For this review, take the finished solid that the model builds, in its own axes (mm). Coordinates: 2 decimals unless noted, no trailing zeros. Write each loop counter-clockwise with the first axis right and the second up, starting at its lowest first coordinate (ties: lowest second). Pieces come first, ordered by that corner, then holes.
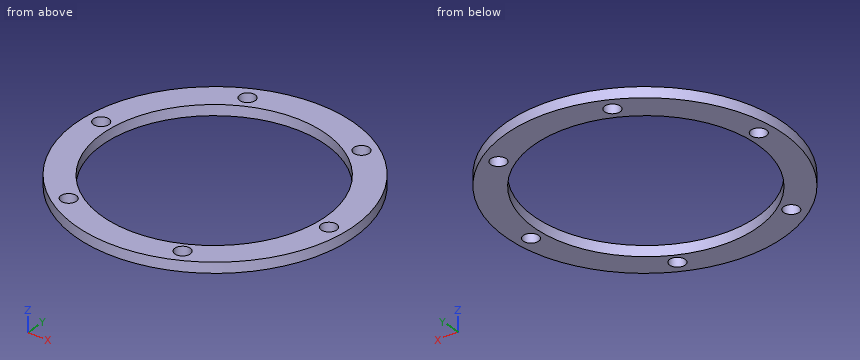
```python
from build123d import *

# Parameters (mm, degrees)
ESQUISSE1_R                  = 30.5
ESQUISSE1_R_2                = 24.5
BOSS_EXTRU_1_DEPTH           = 2.3
ENL_V_MAT_EXTRU_2_REACH      = 45.379
ESQUISSE1_3_R                = 1.7
R_P_TITION_CIRCULAIRE1_COUNT = 6


with BuildPart() as part:
    # Esquisse1 → Boss.-Extru.1 (new body)
    with BuildSketch(Plane.XY):
        with Locations((0, -0.260069897)):
            Circle(ESQUISSE1_R)
        with Locations((0, -0.525514899)):
            Circle(ESQUISSE1_R_2, mode=Mode.SUBTRACT)
    extrude(amount=BOSS_EXTRU_1_DEPTH)

    # Esquisse1_3 → Enl_v. mat.-Extru.2 (cut, up to next)
    with BuildSketch(Plane.XY, mode=Mode.PRIVATE) as enl_v_mat_extru_2_sk1:
        with Locations((15.543281325, 22.122264781)):
            Circle(ESQUISSE1_3_R)
    enl_v_mat_extru_2_tool1 = extrude(enl_v_mat_extru_2_sk1.sketch, amount=ENL_V_MAT_EXTRU_2_REACH, mode=Mode.PRIVATE) & part.part
    enl_v_mat_extru_2 = enl_v_mat_extru_2_tool1.solids().sort_by_distance((15.543281, 22.122265, 0))[0]
    add(enl_v_mat_extru_2, mode=Mode.SUBTRACT)

    # R_p_tition circulaire1: Enl_v. mat.-Extru.2 ×6 about axis
    r_p_tition_circulaire1_axis = Axis((0, -0.260069897, 0), (0, 0, 1))
    for i in range(1, R_P_TITION_CIRCULAIRE1_COUNT):
        add(enl_v_mat_extru_2.rotate(r_p_tition_circulaire1_axis, i * 360 / R_P_TITION_CIRCULAIRE1_COUNT), mode=Mode.SUBTRACT)


solid = part.part
```
Q1. For probe 1 along X at (y, z) = (2, 1.85); probe 2 along X at (y, z) = (-0.5, 0.4); probe 3 along Y at (x, z) = (-11, 1.95), list the stretches that pass through material, from the lowest coordinate up.
Ans:
probe 1: x = -30.42 to -28.86, -25.46 to -24.37, 24.37 to 30.42
probe 2: x = -30.5 to -24.5, 24.5 to 30.5
probe 3: y = -28.71 to -22.42, 21.37 to 22.81, 25.98 to 28.19
Q2. Add section D-D (z = 1.8). State the section outline as (x, y) points.
Ans:
outline: circle Ø61 at (0, -0.26); hole circle Ø3.4 at (-27.16, 2.01); hole circle Ø49 at (0, -0.53); hole circle Ø3.4 at (-15.54, -22.64); hole circle Ø3.4 at (-11.61, 24.39); hole circle Ø3.4 at (11.61, -24.91); hole circle Ø3.4 at (15.54, 22.12); hole circle Ø3.4 at (27.16, -2.53)
Q3. Add section A-A (x = 0). State the section outline as (y, z) points.
Ans:
outline: (-30.76, 0) - (-25.03, 0) - (-25.03, 2.3) - (-30.76, 2.3) - close; (23.97, 0) - (30.24, 0) - (30.24, 2.3) - (23.97, 2.3) - close
Q4. Clearance check with a flat-ended pin moving along its axis: pin 1 Ø2 at (x, y) = (27.16, -2.53) entering from -Z. State where the tip first meets the part, or that it passes through.
Ans:
pin 1: passes through
Q5. Add section B-B (y = -15.5). State the section outline as (x, z) points, then the cut area to 3 significant figures.
Ans:
outline: (-26.42, 0) - (-19.39, 0) - (-19.39, 2.3) - (-26.42, 2.3) - close; (19.39, 0) - (26.42, 0) - (26.42, 2.3) - (19.39, 2.3) - close
area: 32.3 mm2
Q6. Add section C-C (y = -3). State the section outline as (x, z) points.
Ans:
outline: (-30.38, 0) - (-24.37, 0) - (-24.37, 2.3) - (-30.38, 2.3) - close; (24.37, 0) - (25.52, 0) - (25.52, 2.3) - (24.37, 2.3) - close; (28.79, 0) - (30.38, 0) - (30.38, 2.3) - (28.79, 2.3) - close
